Geometry check sheet. Reference: drawing and pictorial views, mm from the part's lowest x, y, z. A direction names the side the tool comes from. Round coordinates to 2 decimals unless told otherwise and drop trailing zeros. Order: outer loops, then holes, each group sorted by start corner. A loop starts at its lowest first (then second) coordinate and runs counter-clockwise, first axis right, second up.
Q1. Cross-section at C-C on z = 5.5. Record the cut outline in (x, y), then the cut area to 3 significant figures.
Q2. Mould release check, pull along X, two halves, no side actions. Record for the marked faces 1, 2 and 3: +X half, -X half, draft (parallel to the pull), parting line (faces both ways), or undercut.
Q3. Cross-section at A-A on z = 7.5. Record the cut outline in (x, y).
Q4. Scan lines: probe 1 along X at (y, z) = (2.5, 8.75); probe 2 along Y at (x, z) = (2.5, 6.5); probe 3 along Z at (x, y) = (7, 0.3). Record each from-to range of solid material in increasing order.
Q5. Set-up check for the marked faces 4, 5 and 6: record each of +Z, -Z, +X, -X, +Y, -Y from which the full face is reachable in a straight line by a thin tool's end or side.
Q6. Depth check by flat-ended pin: P1, Ø1.6, axis at x = 7, z = 5, coming from the -Y side; P2, Ø0.9, axis at x = 2, y = 3, coming from the +Z side. Enter the tip coordinate at first touch or a pass-through.
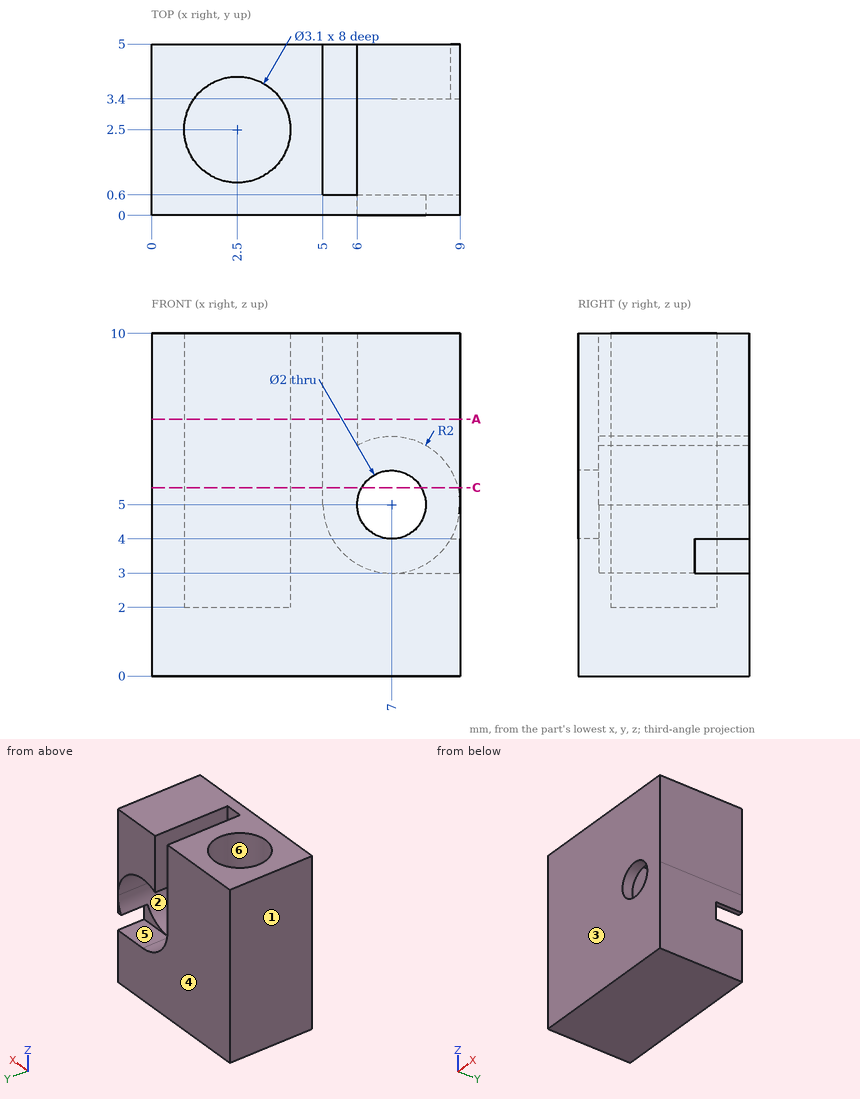
Results found:
1. outline: (0, 0) - (6.13, 0) - (6.13, 0.6) - (5, 0.6) - (5, 5) - (0, 5) - close; (7.87, 0) - (9, 0) - (9, 5) - (8.94, 5) - (8.94, 0.6) - (7.87, 0.6) - close; hole circle Ø3.1 at (2.5, 2.5)
1. area: 19.1 mm2
2. face 1: -X half
2. face 2: undercut
2. face 3: draft
3. outline: (0, 0) - (9, 0) - (9, 5) - (6, 5) - (6, 0.6) - (5, 0.6) - (5, 5) - (0, 5) - close; hole circle Ø3.1 at (2.5, 2.5)
4. probe 1: x = 0 to 0.95, 4.05 to 5, 6 to 9
4. probe 2: y = 0 to 0.95, 4.05 to 5
4. probe 3: z = 0 to 4, 6 to 10
5. face 4: +Z, -Z, +X, -X, +Y
5. face 5: +X, +Y
5. face 6: +Z
6. P1: passes through
6. P2: stops at z = 2
